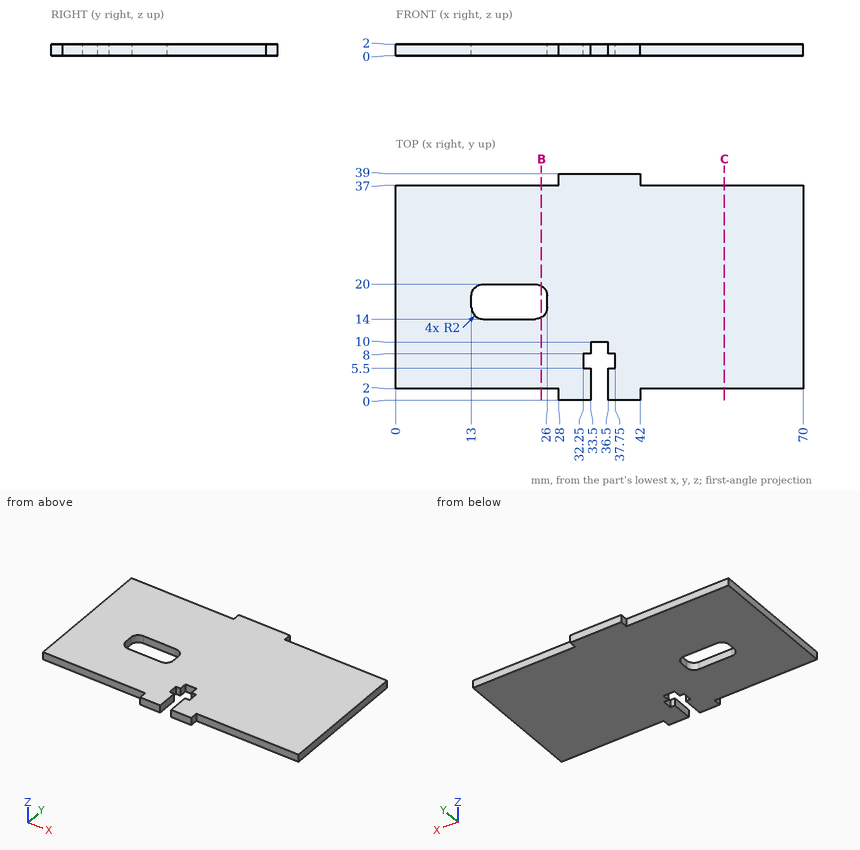
Print and shaded views of the part. All mm, measured from the part's lowest x, y and z. Give positions to 0.01 mm unless a question says otherwise; leave off trailing zeros. Loops run counter-clockwise (first coordinate to the right, second up) from the corner with the lowest first, then second, coordinate; pieces in that order, holes last.
1) Saw through at C-C (x = 56.5). Write the cut outline in (y, z).
2) Wall check: line 1 (X direction, y = 4, z = 1.55); line 2 (X direction, y = 16, z = 1.15); line 3 (Y direction, x = 16.5, z = 0.7). Give the ranges that are in metal, low to high.
3) Flat gauge pins, fed straight in: pin 1 Ø0.6 at (x, z) = (35, 1.5) entering from -Y; pin 2 Ø1 at (x, z) = (53.5, 1) entering from +Y; pin 3 Ø1 at (x, z) = (46.5, 1) entering from -Y; pin 4 Ø1.5 at (x, y) = (45.5, 14.5) entering from -Z. Where does each tip first touch, or does it go through?
4) Saw through at B-B (x = 25). Write the cut outline in (y, z), plus the area to 3 significant figures.
Answer block:
1. outline: (2, 0) - (37, 0) - (37, 2) - (2, 2) - close
2. line 1: x = 0 to 33.5, 36.5 to 70
2. line 2: x = 0 to 13, 26 to 70
2. line 3: y = 2 to 14, 20 to 37
3. pin 1: stops at y = 10
3. pin 2: stops at y = 37
3. pin 3: stops at y = 2
3. pin 4: stops at z = 0
4. outline: (2, 0) - (14.27, 0) - (14.27, 2) - (2, 2) - close; (19.73, 0) - (37, 0) - (37, 2) - (19.73, 2) - close
4. area: 59.1 mm2
